```python
from build123d import *

# Parameters (mm, degrees)
SKETCH_R  = 2.1
PAD_DEPTH = 300
FILLET_R  = 0.4


with BuildPart() as part:
    # Sketch → Pad (new body)
    with BuildSketch(Plane.XY):
        Polygon((-2.84, 3.90066), (2.84, 3.90066), (5.49934, 6.56), (5.49934, 8.2), (3.1, 8.2), (4.9, 10), (10, 10), (10, 4.9), (8.2, 3.1), (8.2, 5.49934), (6.56, 5.49934), (3.90066, 2.84), (3.90066, -2.84), (6.56, -5.49934), (8.2, -5.49934), (8.2, -3.1), (10, -4.9), (10, -10), (4.9, -10), (3.1, -8.2), (5.49934, -8.2), (5.49934, -6.56), (2.84, -3.90066), (-2.84, -3.90066), (-5.49934, -6.56), (-5.49934, -8.2), (-3.1, -8.2), (-4.9, -10), (-10, -10), (-10, -4.9), (-8.2, -3.1), (-8.2, -5.49934), (-6.56, -5.49934), (-3.90066, -2.84), (-3.90066, 2.84), (-6.56, 5.49934), (-8.2, 5.49934), (-8.2, 3.1), (-10, 4.9), (-10, 10), (-4.9, 10), (-3.1, 8.2), (-5.49934, 8.2), (-5.49934, 6.56), align=None)
        Circle(SKETCH_R, mode=Mode.SUBTRACT)
    extrude(amount=PAD_DEPTH)

    # Fillet
    fillet_edges = [part.edges().sort_by_distance(p)[0] for p in [
        (10, 10, 150),
        (-10, 10, 150),
        (10, -10, 150),
        (-10, -10, 150),
    ]]
    fillet(fillet_edges, radius=FILLET_R)


solid = part.part
```
Verification items for the finished model (mm, model axes). A direction names the side the tool comes from. Give positions to 0.01 mm unless a question says otherwise; leave off trailing zeros. Return JSON: item names as keys, results as strings. Group by question number.
1) Scan lines: line 1 (X direction, y = -0.25, z = 262); line 2 (Y direction, x = -8.25, z = 135); line 3 (Y direction, x = 0, z = 238). Record each from-to range of solid material in increasing order.
2) Go/stop test with flat-tipped pins: pin 1 Ø1.5 at (x, z) = (2, 57.5) entering from +Y; pin 2 Ø3 at (y, z) = (0.5, 174) entering from +X; pin 3 Ø0.7 at (x, z) = (4, 219.5) entering from -Y. Record where each tip stops, or that it passes through.
3) Mould release check, pull along Y, two halves, no side actions. Record for faces 4 (the face through (7, -10, 148)), 5 (the face through (3.901, 0, 148)), 6 (the face through (-3.901, 0, 148)), 7 (the face through (10, -7, 148)): pulls with the +Y half, pulls with the -Y half, needs draft (parallel to the pull), parting line crosses it, or undercut.
4) Access from +Z, -Z, +X, -X, +Y, -Y to the whole of each face (thin tool, end or side, straight path). Record for faces 1 (the face through (7, 10, 148)), 2 (the face through (0, 3.901, 148)), 3 (the face through (0, -3.901, 148)).
Answer block:
{
 "1": {"line 1": "x = -3.9 to -2.09, 2.09 to 3.9", "line 2": "y = -10 to -3.15, 3.15 to 10", "line 3": "y = -3.9 to -2.1, 2.1 to 3.9"},
 "2": {"pin 1": "stops at y = 3.9", "pin 2": "stops at x = 3.9", "pin 3": "stops at y = -9.45"},
 "3": {"face 4": "pulls with the -Y half", "face 5": "undercut", "face 6": "undercut", "face 7": "needs draft"},
 "4": {"face 1": "+Z, -Z, +X, -X, +Y", "face 2": "+Z, -Z, +Y", "face 3": "+Z, -Z, -Y"}
}
